Geometry: final body of the model. Coordinates: model frame, mm. Round coordinates to 2 decimals unless told otherwise and drop trailing zeros. Loops run counter-clockwise (first coordinate to the right, second up) from the corner with the lowest first, then second, coordinate; pieces in that order, holes last. Notation, with made-up numbers: (49, -35.75) -> (95, -35.75) arc R35 ccw to (95, 2.25) -> close; hole circle Ø2 at (37.25, 32.25). An arc over 180 degrees is marked (long way). Answer in a Markdown table with one row per item.
```python
from build123d import *

# Parameters (mm, degrees)
SKETCH1_W           = 29.972
SKETCH1_H           = 10.16
BOSS_EXTRUDE1_DEPTH = 86.36
SKETCH2_R           = 1.5875
CUT_EXTRUDE1_DEPTH  = 12.7


with BuildPart() as part:
    # Sketch1 → Boss-Extrude1 (new body)
    with BuildSketch(Plane.XY):
        with Locations((2.823785016, -3.39218241)):
            Rectangle(SKETCH1_W, SKETCH1_H)
    extrude(amount=BOSS_EXTRUDE1_DEPTH)

    # Sketch2 → Cut-Extrude1 (cut)
    with BuildSketch(Plane(origin=(0, 1.68781759, 0), x_dir=(1, 0, 0), z_dir=(0, 1, 0))):
        with Locations(Location((-9.876214984, -8.89, 0), (0, 0, 270))):
            Circle(SKETCH2_R)
        with Locations(Location((15.523785016, -8.89, 0), (0, 0, 270))):
            Circle(SKETCH2_R)
        with Locations(Location((-9.876214984, -77.216, 0), (0, 0, 270))):
            Circle(SKETCH2_R)
        with Locations(Location((15.523785016, -82.296, 0), (0, 0, 270))):
            Circle(SKETCH2_R)
    extrude(amount=-CUT_EXTRUDE1_DEPTH, mode=Mode.SUBTRACT)


solid = part.part
```
Item 1: Mould query, pull axis X, two halves, no side actions, for faces 1 (the flat face through (-12.162, -3, 43)), 2 (the flat face through (3, 1.688, 43)), 3 (the flat face through (17.81, -3, 43)), 4 (the cylindrical face through (-8.8, -3.32, 76.05)). Classes: released by +X, released by -X, zero draft, split by the parting line, or undercut.
Ans:
| item | result |
|---|---|
| face 1 | released by -X |
| face 2 | zero draft |
| face 3 | released by +X |
| face 4 | undercut |
Item 2: Ray query, L1, parallel to X at y = -5.5, z = 8.89; L2, parallel to Z at x = 16.25, y = -1.75; L3, parallel to X at y = -1, z = 76. Return the intervals inside material, ascending.
Ans:
| item | result |
|---|---|
| L1 | -12.16 to -11.46, -8.29 to 13.94, 17.11 to 17.81 |
| L2 | 0 to 7.48, 10.3 to 80.88, 83.71 to 86.36 |
| L3 | -12.16 to -10.9, -8.86 to 17.81 |
Item 3: First-contact query: P1, Ø3, axis at x = 15.52, z = 82.3, coming from the -Y side. Flat tip, straight axial feed; report the tip coordinate or a pass-through.
Ans:
| item | result |
|---|---|
| P1 | through |
Item 4: Section query A-A, the plane z = 8.89. Output: boundary loops of the cut face in (x, y), and give its area (3 significant figures).
Ans:
| item | result |
|---|---|
| outline | (-12.16, -8.47) -> (-11.46, -8.47) -> (-11.46, 1.69) -> (-12.16, 1.69) -> close; (-8.29, -8.47) -> (13.94, -8.47) -> (13.94, 1.69) -> (-8.29, 1.69) -> close; (17.11, -8.47) -> (17.81, -8.47) -> (17.81, 1.69) -> (17.11, 1.69) -> close |
| area | 240 mm2 |
Item 5: Section query B-B, the plane z = 77. Output: boundary loops of the cut face in (x, y), and give its area (3 significant figures).
Ans:
| item | result |
|---|---|
| outline | (-12.16, -8.47) -> (-11.45, -8.47) -> (-11.45, 1.69) -> (-12.16, 1.69) -> close; (-8.3, -8.47) -> (17.81, -8.47) -> (17.81, 1.69) -> (-8.3, 1.69) -> close |
| area | 273 mm2 |
